The model under review builds one solid part; all positions refer to its coordinate system, in mm. A direction names the side the tool comes from. Round coordinates to 2 decimals unless told otherwise and drop trailing zeros. Order: outer loops, then holes, each group sorted by start corner. A loop starts at its lowest first (then second) coordinate and runs counter-clockwise, first axis right, second up. Notation, with made-up numbers: M 66.25,85.25 L 72.25,85.25 A30 ccw 72.25,114.25 Z; hole C -24,24.5 d1. An arc over 180 degrees is marked long. Use a Markdown table: item, result. Add a question column.
1. Consider section A-A on z = -2.05. State the section outline as (x, y) points, then the cut area to 3 significant figures.
2. For faces 1 (the flat face through (3.15, -1.85, 0)), 2 (the cylindrical face through (3.233, 1.341, 0.197)), 3 (the flat face through (-3.2, 1.9, 0)), 4 (the flat face through (3.15, 1.86, 0)), 5 (the flat face through (0, -3.7, 0)), list the 3-axis set-ups (+Z, -Z, +X, -X, +Y, -Y) from which the entire face can be reached by the end or side of a thin tool; tool diameter is ignored.
3. Insertion check: P1, Ø1.9, axis at x = 3, y = 2, coming from the +Z side; P2, Ø1, axis at x = -1, z = -0.5, coming from the +Y side. Each pin has a flat end and moves straight along its axis. Give the tip position at first contact, or say it passes through.
4. Consider section B-B on y = -3.25. State the section outline as (x, z) points, then the cut area to 3 significant figures.
5. To check wall thickness, follow probe 1 along Y at (x, z) = (-1, -0.4); probe 2 along X at (y, z) = (-0.75, -0.2); probe 3 along X at (y, z) = (1, -0.9). State the ranges of each line that lie inside material, in increasing order.
6. The part is to be moulded in two halves that separate along X. For faces 6 (the cylindrical face through (-1.216, -1.115, -1.218)), 7 (the flat face through (-3.2, -1.8, 0)), 8 (the flat face through (1.725, 3.045, -1.38)), say which applies: +X half, -X half, draft (parallel to the pull), parting line (faces both ways), or undercut.
Autodesk Inventor part; units mm, degrees
ref_plane "YZ Plane" through (0, 0, 0) normal (1, 0, 0) x (0, 1, 0)
ref_plane "XZ Plane" through (0, 0, 0) normal (0, 1, 0) x (-1, 0, 0)
ref_plane "XY Plane" through (0, 0, 0) normal (0, 0, 1) x (1, 0, 0)
sketch "Szkic1" plane through (0, 0, 0) normal (0, 0, 1) x (1, 0, 0)
  circle A0 centre (0, 0) radius 3.5
  circle A1 centre (0, 0) radius 1.65
  dimension "d0" = 7
  dimension "d1" = 3.3
extrude "Wyciągnięcie proste1" add sketch "Szkic1" along normal blind 0.4
chamfer "Faza1" distance 0.35 angle 45 1 edges at (-1.65, 0, 0.4)
sketch "Szkic2" plane through (0, 0, 0.4) normal (0, 0, 1) x (1, 0, 0)
  point P0 (0, 0)
sketch "Szkic3" plane through (0, 0, 0) normal (0, 0, -1) x (-1, 0, 0)
  circle A0 centre (0, 0) radius 1.65
  circle A1 centre (0, 0) radius 3.5
  circle A2 centre (0, 0) radius 3.5
  line L0 (1.75, 3.0311) -> (3.5, 2.0207)
  line L1 (1.75, 3.0311) -> (0, 4.0415)
  line L2 (-1.75, 3.0311) -> (0, 4.0415)
  line L3 (-1.75, 3.0311) -> (-3.5, 2.0207)
  line L4 (-3.5, 0) -> (-3.5, 2.0207)
  line L5 (-3.5, 0) -> (-3.5, -2.0207)
  line L6 (-1.75, -3.0311) -> (-3.5, -2.0207)
  line L7 (-1.75, -3.0311) -> (0, -4.0415)
  line L8 (0, -4.0415) -> (1.75, -3.0311)
  line L9 (1.75, -3.0311) -> (3.5, -2.0207)
  line L10 (3.5, 0) -> (3.5, -2.0207)
  line L11 (3.5, 0) -> (3.5, 2.0207)
extrude "Wyciągnięcie proste2" add sketch "Szkic3" along normal blind 2.8 contours A0 | A1 | L10 L9 A1 | A1 L0 L11 | A1 L2 L1 | L8 L7 A1 | A1 L4 L3 | L6 L5 A1
sketch "Szkic4" plane through (0, 0, 0) normal (0, 0, 1) x (1, 0, 0)
  circle A0 centre (0, 0) radius 1.65
extrude "Wyciągnięcie proste3" cut sketch "Szkic4" against normal blind 2.8
chamfer "Faza2" distance 0.35 angle 45 1 edges at (-1.65, 0, -2.8)
sketch "Szkic5" plane through (0, 0, -2.8) normal (0, 0, -1) x (-1, 0, 0)
  circle A0 centre (0, 0) radius 3.5
  dimension "d18" = 7
sketch "Szkic6" plane through (0, 0, -2.8) normal (0, 0, -1) x (-1, 0, 0)
  line L0 (-3.5, 2.0207) -> (-3.5, -2.0207)
  line L1 (-3.5, -2.0207) -> (-3.5, 0)
  line L2 (-3.5, 2.0207) -> (-3.5, 0)
  line L3 (-3.5, 0) -> (-3.5, 2.0207)
  line L4 (-3.5, 2.0207) -> (-1.75, 3.0311)
  line L5 (0, 4.0415) -> (-3.5, 2.0207)
  line L6 (-1.75, 3.0311) -> (0, 4.0415)
  line L7 (0, 4.0415) -> (1.75, 3.0311)
  line L8 (3.5, 2.0207) -> (0, 4.0415)
  line L9 (1.75, 3.0311) -> (3.5, 2.0207)
  line L10 (3.5, 2.0207) -> (3.5, 0)
  line L11 (3.5, -2.0207) -> (3.5, 0)
  line L12 (3.5, 0) -> (3.5, -2.0207)
  arc A0 (-1.75, -3.0311) -> (1.75, -3.0311) centre (0, 0) ccw
  line L13 (3.5, -2.0207) -> (1.75, -3.0311)
  line L14 (-3.5, -2.0207) -> (0, -4.0415)
  line L15 (1.75, -3.0311) -> (0, -4.0415)
  line L16 (0, -4.0415) -> (-1.75, -3.0311)
  arc A1 (-3.5, 0) -> (-1.75, -3.0311) centre (0, 0) ccw
  line L17 (-1.75, -3.0311) -> (-3.5, -2.0207)
sketch "Szkic7" plane through (0, 0, -2.8) normal (0, 0, -1) x (-1, 0, 0)
  point P0 (0, 0)
properties part number "nakretka"
Answer block:
| question | item | result |
|---|---|---|
| 1 | outline | M -3.5,-2.02 L 0,-4.04 L 3.5,-2.02 L 3.5,2.02 L 0,4.04 L -3.5,2.02 Z; hole C 0,0 d3.3 |
| 1 | area | 33.9 mm^2 |
| 2 | face 1 | +Z, +X, -Y |
| 2 | face 2 | +Z |
| 2 | face 3 | +Z, -X, +Y |
| 2 | face 4 | +Z, +X, +Y |
| 2 | face 5 | +Z, -Y |
| 3 | P1 | z = 0.4 |
| 3 | P2 | y = 3.75 |
| 4 | outline | M -1.37,-2.8 L 1.37,-2.8 L 1.37,0 L 1.3,0 L 1.3,0.4 L -1.3,0.4 L -1.3,0 L -1.37,0 Z |
| 4 | area | 8.72 mm^2 |
| 5 | probe 1 | -3.46 to -1.31, 1.31 to 3.46 |
| 5 | probe 2 | -3.5 to -1.47, 1.47 to 3.5 |
| 5 | probe 3 | -3.5 to -1.31, 1.31 to 3.5 |
| 6 | face 6 | undercut |
| 6 | face 7 | draft |
| 6 | face 8 | +X half |
